Input: part model. Units: mm. Frame: model coordinates. A direction names the side the tool comes from. Round coordinates to 2 decimals unless told otherwise and drop trailing zeros. Loops run counter-clockwise (first coordinate to the right, second up) from the corner with the lowest first, then second, coordinate; pieces in that order, holes last.
1) First-contact query: pin 1 (5 mm diameter, centred on x = -33.5, y = -8.5, fed in from -Z); pin 2 (2.5 mm diameter, centred on x = 77.79, y = -22.78, fed in from -Z). Flat tips, straight axial feed; report the tip coordinate or a pass-through.
2) Section B-B, the plane z = 1.35. State how many separate pieces and enclosed holes the cut face has, and give its area (3 significant figures).
3) Draft query along X for faces 1 (the face through (-27.21, 15.95, 1.57)), 2 (the face through (-82.55, -20, 2)), 3 (the face through (-1, -58.337, 2)). Return one class per face: pulls with the +X half, pulls with the -X half, needs draft (parallel to the pull), parting line crosses it, or undercut.
4) Section D-D, the plane x = -14.5. Return loops of the section in (y, z) (3 decimals), and give its area (3 significant figures).
5) Section A-A, the plane x = 63.5. Return loops of the section in (y, z) (3 decimals), and give its area (3 significant figures).
6) Access query for faces 4 (the face through (11.003, -41.148, 1.565)), 5 (the face through (-25.4, 7, 2)). Directions: +Z, -Z, +X, -X, +Y, -Y. A direction counts if a zero-diameter tool reaches every point of the face in a straight line with its end or side. Return the directions, or none.
7) Ray query, line 1 along X through (y, z) = (-22.5, 2.8); line 2 along Y through (x, z) = (63.5, 0.8); line 3 along X through (y, z) = (8, 1.8). Return the intervals inside material, ascending.
8) Section C-C, the plane x = 11. Return loops of the section in (y, z) (3 decimals).
from build123d import *

# Parameters (mm, degrees)
SKETCH5_R           = 1.5875
SKETCH5_R_2         = 1.906243542
BOSS_EXTRUDE2_DEPTH = 3.175


with BuildPart() as part:
    # Sketch5 → Boss-Extrude2 (new body)
    with BuildSketch(Plane.XY):
        with BuildLine():
            Line((-82.55, 17.863023715), (-82.55, -58.336976285))
            Line((-82.55, -58.336976285), (82.55, -58.336976285))
            Line((82.55, -58.336976285), (82.55, 17.863023715))
            Line((82.55, 17.863023715), (31.75, 17.863023715))
            ThreePointArc((31.75, 17.863023715), (27.259871939, 16.003151775), (25.4, 11.513023715))
            Line((25.4, 11.513023715), (25.4, 1.988023715))
            ThreePointArc((25.4, 1.988023715), (24.47006403, -0.257040316), (22.225, -1.186976285))
            Line((22.225, -1.186976285), (-22.225, -1.186976285))
            ThreePointArc((-22.225, -1.186976285), (-24.47006403, -0.257040316), (-25.4, 1.988023715))
            Line((-25.4, 1.988023715), (-25.4, 11.513023715))
            ThreePointArc((-25.4, 11.513023715), (-27.259871939, 16.003151775), (-31.75, 17.863023715))
            Line((-31.75, 17.863023715), (-82.55, 17.863023715))
        make_face()
        with Locations((-77.7875, -40.556976285)):
            Circle(SKETCH5_R, mode=Mode.SUBTRACT)
        with Locations((-77.7875, -22.776976285)):
            Circle(SKETCH5_R, mode=Mode.SUBTRACT)
        with Locations((-77.7875, -4.996976285)):
            Circle(SKETCH5_R, mode=Mode.SUBTRACT)
        with Locations((-77.7875, 12.783023715)):
            Circle(SKETCH5_R, mode=Mode.SUBTRACT)
        with Locations((11.416585625, -39.286976285)):
            Circle(SKETCH5_R_2, mode=Mode.SUBTRACT)
        with Locations((63.5, -39.286976285)):
            Circle(SKETCH5_R_2, mode=Mode.SUBTRACT)
        with Locations((77.7875, 12.783023715)):
            Circle(SKETCH5_R, mode=Mode.SUBTRACT)
        with Locations((77.7875, -4.996976285)):
            Circle(SKETCH5_R, mode=Mode.SUBTRACT)
        with Locations((77.7875, -22.776976285)):
            Circle(SKETCH5_R, mode=Mode.SUBTRACT)
        with Locations((77.7875, -40.556976285)):
            Circle(SKETCH5_R, mode=Mode.SUBTRACT)
    extrude(amount=BOSS_EXTRUDE2_DEPTH)


solid = part.part
Final values:
1. pin 1: stops at z = 0
1. pin 2: passes through
2. separate pieces: 1
2. enclosed holes: 10
2. area: 11,500 mm2
3. face 1: undercut
3. face 2: pulls with the -X half
3. face 3: needs draft
4. outline: (-58.337, 0) - (-1.187, 0) - (-1.187, 3.175) - (-58.337, 3.175) - close
4. area: 181 mm2
5. outline: (-58.337, 0) - (-41.193, 0) - (-41.193, 3.175) - (-58.337, 3.175) - close; (-37.381, 0) - (17.863, 0) - (17.863, 3.175) - (-37.381, 3.175) - close
5. area: 230 mm2
6. face 4: +Z, -Z
6. face 5: +Z, -Z, +Y
7. line 1: x = -82.55 to -79.35, -76.22 to 76.22, 79.35 to 82.55
7. line 2: y = -58.34 to -41.19, -37.38 to 17.86
7. line 3: x = -82.55 to -25.4, 25.4 to 82.55
8. outline: (-58.337, 0) - (-41.147, 0) - (-41.147, 3.175) - (-58.337, 3.175) - close; (-37.427, 0) - (-1.187, 0) - (-1.187, 3.175) - (-37.427, 3.175) - close
